```python
from build123d import *

# Parameters (mm, degrees)
F0_R     = 12.5
F1_DEPTH = 8


with BuildPart() as f1:
    # F0 (on Top) → F1 (new body)
    with BuildSketch(Plane.XY):
        with BuildLine():
            ThreePointArc((0, 17.5), (5.125631, 5.125631), (17.5, 0))
            Line((17.5, 0), (81, 0))
            ThreePointArc((81, 0), (84.535534, 1.464466), (86, 5))
            Line((86, 5), (86, 30))
            ThreePointArc((86, 30), (84.535534, 33.535534), (81, 35))
            Line((81, 35), (17.5, 35))
            ThreePointArc((17.5, 35), (5.125631, 29.874369), (0, 17.5))
        make_face()
        with Locations((17.5, 17.5)):
            Circle(F0_R, mode=Mode.SUBTRACT)
    extrude(amount=F1_DEPTH)

    # F2 (on face) → F3 (revolve, cut)
    with BuildSketch(Plane.XY.offset(8)):
        with BuildLine():
            Line((41, 23), (41, 7))
            Line((41, 7), (42, 7))
            Line((42, 7), (44, 10))
            Line((44, 10), (44, 23))
            Line((44, 23), (47.25, 23))
            Line((47.25, 23), (47.25, 24.5))
            ThreePointArc((47.25, 24.5), (46.517767, 26.267767), (44.75, 27))
            Line((44.75, 27), (41, 27))
            Line((41, 27), (41, 23))
        make_face()
    revolve(axis=Axis((41, 15, 8), (0, 1, 0)), mode=Mode.SUBTRACT)

    # F2 (on face) → F4 (revolve, cut)
    with BuildSketch(Plane.XY.offset(8)):
        with BuildLine():
            Line((58.5, 23), (58.5, 7))
            Line((58.5, 7), (59.5, 7))
            Line((59.5, 7), (61.5, 10))
            Line((61.5, 10), (61.5, 23))
            Line((61.5, 23), (64.75, 23))
            Line((64.75, 23), (64.75, 24.5))
            ThreePointArc((64.75, 24.5), (64.017767, 26.267767), (62.25, 27))
            Line((62.25, 27), (58.5, 27))
            Line((58.5, 27), (58.5, 23))
        make_face()
    revolve(axis=Axis((58.5, 15, 8), (0, 1, 0)), mode=Mode.SUBTRACT)

    # F2 (on face) → F5 (revolve, cut)
    with BuildSketch(Plane.XY.offset(8)):
        with BuildLine():
            Line((76, 23), (76, 7))
            Line((76, 7), (77, 7))
            Line((77, 7), (79, 10))
            Line((79, 10), (79, 23))
            Line((79, 23), (82.25, 23))
            Line((82.25, 23), (82.25, 24.5))
            ThreePointArc((82.25, 24.5), (81.517767, 26.267767), (79.75, 27))
            Line((79.75, 27), (76, 27))
            Line((76, 27), (76, 23))
        make_face()
    revolve(axis=Axis((76, 15, 8), (0, 1, 0)), mode=Mode.SUBTRACT)


solid = f1.part
```
Here's how the part is built. I have some questions about the finished solid (model axes, mm). A direction names the side the tool comes from. Give positions to 0.01 mm unless a question says otherwise; leave off trailing zeros. Write each loop counter-clockwise with the first axis right and the second up, starting at its lowest first coordinate (ties: lowest second). Pieces come first, ordered by that corner, then holes. Notation, with made-up numbers: (56, -3.5) -> (100, -3.5) arc R8 ccw to (100, 4.5) -> close; hole circle Ø2 at (4, 88). An arc over 180 degrees is marked (long way). Use one line per item in the form item = value.
1) I'm going to push flat-ended pins straight in: pin 1 (12 mm diameter, centred on x = 76.5, y = 11.5, fed in from +Z); pin 2 (1 mm diameter, centred on x = 13.5, z = 4.5, fed in from -Y); pin 3 (15 mm diameter, centred on x = 17.5, y = 17.5, fed in from +Z); pin 4 (1 mm diameter, centred on y = 31, z = 3, fed in from +X). Where does each tip first touch, or does it pass through?
Verdict:
pin_1 = 8
pin_2 = 0.35
pin_3 = through
pin_4 = 85.97
2) On a 3-axis mill with a long thin cutter (end or side, diameter ignored), from which of +Z, -Z, +X, -X, +Y, -Y can I reach the whole of each face in a straight line? I mean faces 1 (the face through (58.64, 23.76, 1.75)), 2 (the face through (85, 33, 4)). Say none if no direction works.
Verdict:
face_1 = +Z
face_2 = +Z, -Z, +X, +Y
3) If I drill on L1, parallel to Y at x = 75, z = 4.25; L2, parallel to Y at x = 17.5, z = 5.75; L3, parallel to X at y = 12, z = 5.25, over which ranges is the centre line in solid material (lowest first)? Write a range as [from, to].
Verdict:
L1 = [0, 23], [27, 35]
L2 = [0, 5], [30, 35]
L3 = [0.89, 6.28], [28.72, 39.8], [42.2, 57.3], [59.7, 74.8], [77.2, 86]
4) Suppose I cut it at B-B (y = 11.5). Please give me the cut outline in (x, z).
Verdict:
outline = (1.06, 0) -> (6.53, 0) -> (6.53, 8) -> (1.06, 8) -> close; (28.47, 0) -> (86, 0) -> (86, 8) -> (79, 8) arc R3 cw to (73, 8) -> (61.5, 8) arc R3 cw to (55.5, 8) -> (44, 8) arc R3 cw to (38, 8) -> (28.47, 8) -> close
5) Suppose I cut it at A-A (x = 76). Please give me the cut outline in (y, z).
Verdict:
outline = (0, 0) -> (35, 0) -> (35, 8) -> (27, 8) -> (27, 4.25) arc R2.5 cw to (24.5, 1.75) -> (23, 1.75) -> (23, 5) -> (10, 5) -> (7, 7) -> (7, 8) -> (0, 8) -> close
6) Suppose I cut it at D-D (y = 28). Please give me the cut outline in (x, z).
Verdict:
outline = (3.5, 0) -> (10.72, 0) -> (10.72, 8) -> (3.5, 8) -> close; (24.28, 0) -> (86, 0) -> (86, 8) -> (24.28, 8) -> close
7) We'd pull the mould along Y, two halves only. Please class faces 3 (the face through (50, 35, 4)), 4 (the face through (49, 0, 4)), 5 (the face through (76, 17, 5)): +Y half, -Y half, draft (parallel to the pull), parting line (faces both ways), or undercut.
Verdict:
face_3 = +Y half
face_4 = -Y half
face_5 = undercut
8) Suppose I cut it at C-C (x = 7). Please give me the cut outline in (y, z), and give its area (3 significant figures).
Verdict:
outline = (3.5, 0) -> (10.72, 0) -> (10.72, 8) -> (3.5, 8) -> close; (24.28, 0) -> (31.5, 0) -> (31.5, 8) -> (24.28, 8) -> close
area = 115 mm2
